Check sheet for the modelled part. Datum: model origin and axes. Units: mm. A direction names the side the tool comes from. Round coordinates to 2 decimals unless told otherwise and drop trailing zeros. Order: outer loops, then holes, each group sorted by start corner. A loop starts at its lowest first (then second) coordinate and runs counter-clockwise, first axis right, second up. Notation, with made-up numbers: M 7.5,9.25 L 65.5,9.25 A18 ccw 65.5,22.25 Z; hole C -25,-34.75 d4. An arc over 180 degrees is marked long. One line per item, written item: value. Start each with the question number.
(1) Release check for a two-part mould opening along Z. For faces 1 (the face through (25, 1, 0)), 2 (the face through (42, 2, 16.499)), 3 (the face through (32.302, 0.74, 1.462)) record: released by +Z, released by -Z, zero draft, split by the parting line, or undercut.
(2) Cross-section at D-D, the plane z = 13.25. Enter the section's corners in (x, y), and give its area (3 significant figures).
(3) Cross-section at B-B, the plane x = 39.46. Enter the section's corners in (y, z), and give its area (3 significant figures).
(4) Cross-section at A-A, the plane y = 3. Enter the section's corners in (x, z).
(5) Depth check by flat-ended pin: pin 1 Ø8 at (x, z) = (38.5, 9.5) entering from +Y; pin 2 Ø2 at (x, y) = (41.5, 4) entering from -Z; pin 3 Ø12 at (x, z) = (27.5, 4) entering from +Y. Enter the tip coordinate at first touch or a pass-through.
(6) Cross-section at C-C, the plane x = 11.52. Enter the section's corners in (y, z), and give its area (3 significant figures).
(7) Thickness scan on L1, parallel to Z at x = 44.54, y = 1.2; L2, parallel to Y at x = 47.5, z = 14.25; L3, parallel to Z at x = 48.5, y = 2.75. Record the ranges inside material, lowest first.
(8) Access from +Z, -Z, +X, -X, +Y, -Y to the whole of each face (thin tool, end or side, straight path). Record for faces 4 (the face through (48.118, 3, 11)), 5 (the face through (24, 2.25, 12)), 6 (the face through (48.81, 1.99, 15.18)).
from build123d import *

# Parameters (mm, degrees)
SKETCH1_R           = 0.5
SKETCH1_R_2         = 1.5
BOSS_EXTRUDE1_DEPTH = 1.5
SKETCH3_W           = 13.585431646
SKETCH3_H           = 8.151258988
BOSS_EXTRUDE2_DEPTH = 2.5
SKETCH4_W           = 1.964423464
SKETCH4_H           = 7.620608266
BOSS_EXTRUDE3_DEPTH = 3
SKETCH5_W           = 18.269857108
SKETCH5_H           = 9.951352814
SKETCH5_R           = 0.457577412
BOSS_EXTRUDE4_DEPTH = 1
SKETCH6_W           = 7.030512295
SKETCH6_H           = 7.030512295
BOSS_EXTRUDE5_DEPTH = 0.75


with BuildPart() as part:
    # Sketch1 → Boss-Extrude1 (new body)
    with BuildSketch(Plane(origin=(0, 0, 0), x_dir=(1, 0, 0), z_dir=(0, 1, 0))):
        with BuildLine():
            Line((2.63, 0), (48.35, 0))
            ThreePointArc((48.35, 0), (50.209690835, -0.770309165), (50.98, -2.63))
            Line((50.98, -2.63), (50.98, -20.23))
            ThreePointArc((50.98, -20.23), (50.209690835, -22.089690835), (48.35, -22.86))
            Line((48.35, -22.86), (2.63, -22.86))
            ThreePointArc((2.63, -22.86), (0.770309165, -22.089690835), (0, -20.23))
            Line((0, -20.23), (0, -2.63))
            ThreePointArc((0, -2.63), (0.770309165, -0.770309165), (2.63, 0))
        make_face()
        with Locations((6.44, -21.59)):
            Circle(SKETCH1_R, mode=Mode.SUBTRACT)
        with Locations((8.98, -21.59)):
            Circle(SKETCH1_R, mode=Mode.SUBTRACT)
        with Locations((11.52, -21.59)):
            Circle(SKETCH1_R, mode=Mode.SUBTRACT)
        with Locations((14.06, -21.59)):
            Circle(SKETCH1_R, mode=Mode.SUBTRACT)
        with Locations((16.6, -21.59)):
            Circle(SKETCH1_R, mode=Mode.SUBTRACT)
        with Locations((19.14, -21.59)):
            Circle(SKETCH1_R, mode=Mode.SUBTRACT)
        with Locations((21.68, -21.59)):
            Circle(SKETCH1_R, mode=Mode.SUBTRACT)
        with Locations((24.22, -21.59)):
            Circle(SKETCH1_R, mode=Mode.SUBTRACT)
        with Locations((26.76, -21.59)):
            Circle(SKETCH1_R, mode=Mode.SUBTRACT)
        with Locations((29.3, -21.59)):
            Circle(SKETCH1_R, mode=Mode.SUBTRACT)
        with Locations((31.84, -21.59)):
            Circle(SKETCH1_R, mode=Mode.SUBTRACT)
        with Locations((34.38, -21.59)):
            Circle(SKETCH1_R, mode=Mode.SUBTRACT)
        with Locations((36.92, -21.59)):
            Circle(SKETCH1_R, mode=Mode.SUBTRACT)
        with Locations((39.46, -21.59)):
            Circle(SKETCH1_R, mode=Mode.SUBTRACT)
        with Locations((42, -21.59)):
            Circle(SKETCH1_R, mode=Mode.SUBTRACT)
        with Locations((44.54, -21.59)):
            Circle(SKETCH1_R, mode=Mode.SUBTRACT)
        with Locations((44.54, -1.27)):
            Circle(SKETCH1_R, mode=Mode.SUBTRACT)
        with Locations((42, -1.27)):
            Circle(SKETCH1_R, mode=Mode.SUBTRACT)
        with Locations((39.46, -1.27)):
            Circle(SKETCH1_R, mode=Mode.SUBTRACT)
        with Locations((36.92, -1.27)):
            Circle(SKETCH1_R, mode=Mode.SUBTRACT)
        with Locations((34.38, -1.27)):
            Circle(SKETCH1_R, mode=Mode.SUBTRACT)
        with Locations((31.84, -1.27)):
            Circle(SKETCH1_R, mode=Mode.SUBTRACT)
        with Locations((29.3, -1.27)):
            Circle(SKETCH1_R, mode=Mode.SUBTRACT)
        with Locations((26.76, -1.27)):
            Circle(SKETCH1_R, mode=Mode.SUBTRACT)
        with Locations((24.22, -1.27)):
            Circle(SKETCH1_R, mode=Mode.SUBTRACT)
        with Locations((21.68, -1.27)):
            Circle(SKETCH1_R, mode=Mode.SUBTRACT)
        with Locations((19.14, -1.27)):
            Circle(SKETCH1_R, mode=Mode.SUBTRACT)
        with Locations((16.6, -1.27)):
            Circle(SKETCH1_R, mode=Mode.SUBTRACT)
        with Locations((2.63, -2.54)):
            Circle(SKETCH1_R_2, mode=Mode.SUBTRACT)
        with Locations((2.63, -20.32)):
            Circle(SKETCH1_R_2, mode=Mode.SUBTRACT)
        with Locations((48.35, -20.32)):
            Circle(SKETCH1_R_2, mode=Mode.SUBTRACT)
        with Locations((48.35, -2.54)):
            Circle(SKETCH1_R_2, mode=Mode.SUBTRACT)
    extrude(amount=BOSS_EXTRUDE1_DEPTH)

    # Sketch3 → Boss-Extrude2 (add)
    with BuildSketch(Plane(origin=(0, 1.5, 0), x_dir=(1, 0, 0), z_dir=(0, 1, 0))):
        with Locations((40.399579876, -11.65885309)):
            Rectangle(SKETCH3_W, SKETCH3_H)
    extrude(amount=BOSS_EXTRUDE2_DEPTH)

    # Sketch4 → Boss-Extrude3 (add)
    with BuildSketch(Plane(origin=(0, 1.5, 0), x_dir=(1, 0, 0), z_dir=(0, 1, 0))):
        with Locations((49.100080702, -10.717871328)):
            Rectangle(SKETCH4_W, SKETCH4_H)
    extrude(amount=BOSS_EXTRUDE3_DEPTH)

    # Sketch5 → Boss-Extrude4 (add)
    with BuildSketch(Plane(origin=(0, 1.5, 0), x_dir=(1, 0, 0), z_dir=(0, 1, 0))):
        with Locations((41.845071446, -11.523458661)):
            Rectangle(SKETCH5_W, SKETCH5_H)
        with Locations((48.865489617, -15.632765099)):
            Circle(SKETCH5_R, mode=Mode.SUBTRACT)
    extrude(amount=BOSS_EXTRUDE4_DEPTH)

    # Sketch6 → Boss-Extrude5 (add)
    with BuildSketch(Plane(origin=(0, 1.5, 0), x_dir=(1, 0, 0), z_dir=(0, 1, 0))):
        with Locations((23.761662883, -11.839547187)):
            Rectangle(SKETCH6_W, SKETCH6_H)
    extrude(amount=BOSS_EXTRUDE5_DEPTH)


solid = part.part
Values found:
1. face 1: released by -Z
1. face 2: released by +Z
1. face 3: undercut
2. outline: M 0,0 L 50.98,0 L 50.98,2.5 L 50.08,2.5 L 50.08,4.5 L 48.12,4.5 L 48.12,2.5 L 47.19,2.5 L 47.19,4 L 33.61,4 L 33.61,2.5 L 32.71,2.5 L 32.71,1.5 L 27.28,1.5 L 27.28,2.25 L 20.25,2.25 L 20.25,1.5 L 0,1.5 Z
2. area: 124 mm^2
3. outline: M 0,0 L 1.5,0 L 1.5,0.77 L 0,0.77 Z; M 0,1.77 L 1.5,1.77 L 1.5,6.55 L 2.5,6.55 L 2.5,7.58 L 4,7.58 L 4,15.73 L 2.5,15.73 L 2.5,16.5 L 1.5,16.5 L 1.5,21.09 L 0,21.09 Z; M 0,22.09 L 1.5,22.09 L 1.5,22.86 L 0,22.86 Z
3. area: 53.5 mm^2
4. outline: M 33.61,7.58 L 47.19,7.58 L 47.19,15.73 L 33.61,15.73 Z; M 48.12,6.91 L 50.08,6.91 L 50.08,14.53 L 48.12,14.53 Z
5. pin 1: y = 4
5. pin 2: z = 7.58
5. pin 3: y = 2.5
6. outline: M 0,0 L 1.5,0 L 1.5,21.09 L 0,21.09 Z; M 0,22.09 L 1.5,22.09 L 1.5,22.86 L 0,22.86 Z
6. area: 32.8 mm^2
7. L1: 0 to 0.77, 1.77 to 21.09, 22.09 to 22.86
7. L2: 0 to 2.5
7. L3: 6.91 to 14.53
8. face 4: +Z, -Z, +Y
8. face 5: +Z, -Z, -X, +Y
8. face 6: +Y
